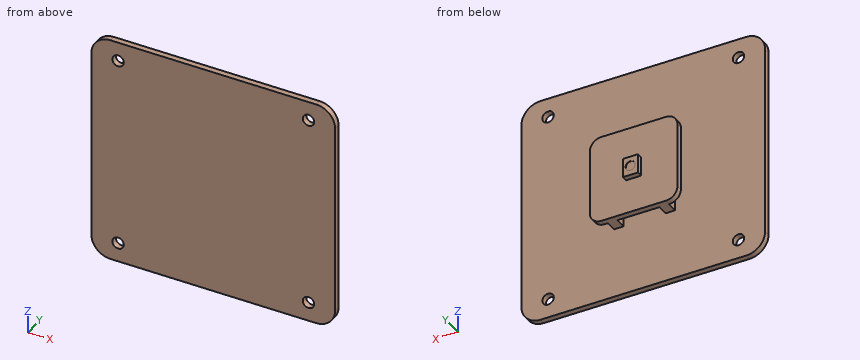
from build123d import *

# Parameters (mm, degrees)
SKETCH1_R           = 1.5
BOSS_EXTRUDE1_DEPTH = 1.6
SKETCH2_W           = 23
SKETCH2_H           = 23
BOSS_EXTRUDE2_DEPTH = 4.5
SKETCH3_W           = 4
SKETCH3_H           = 5
BOSS_EXTRUDE3_DEPTH = 1.5
SKETCH4_W           = 23
SKETCH4_H           = 2.9
CUT_EXTRUDE3_DEPTH  = 39.5
SKETCH5_W           = 2.5
SKETCH5_H           = 2.9
BOSS_EXTRUDE4_DEPTH = 23
FILLET1_R           = 3
SKETCH6_R           = 1.25
CUT_EXTRUDE4_DEPTH  = 0.1


with BuildPart() as part:
    # Sketch1 → Boss-Extrude1 (new body)
    with BuildSketch(Plane(origin=(0, 0, 0), x_dir=(1, 0, 0), z_dir=(0, 1, 0))):
        with BuildLine():
            Line((-27, -30), (27, -30))
            ThreePointArc((27, -30), (30.535533906, -28.535533906), (32, -25))
            Line((32, -25), (32, 25))
            ThreePointArc((32, 25), (30.535533906, 28.535533906), (27, 30))
            Line((27, 30), (-27, 30))
            ThreePointArc((-27, 30), (-30.535533906, 28.535533906), (-32, 25))
            Line((-32, 25), (-32, -25))
            ThreePointArc((-32, -25), (-30.535533906, -28.535533906), (-27, -30))
        make_face()
        with Locations((25, 25)):
            Circle(SKETCH1_R, mode=Mode.SUBTRACT)
        with Locations((-25, 25)):
            Circle(SKETCH1_R, mode=Mode.SUBTRACT)
        with Locations((-25, -25)):
            Circle(SKETCH1_R, mode=Mode.SUBTRACT)
        with Locations((25, -25)):
            Circle(SKETCH1_R, mode=Mode.SUBTRACT)
    extrude(amount=BOSS_EXTRUDE1_DEPTH)

    # Sketch2 → Boss-Extrude2 (add)
    with BuildSketch(Plane(origin=(0, 1.6, 0), x_dir=(1, 0, 0), z_dir=(0, 1, 0))):
        Rectangle(SKETCH2_W, SKETCH2_H)
    extrude(amount=BOSS_EXTRUDE2_DEPTH)

    # Sketch3 → Boss-Extrude3 (add)
    with BuildSketch(Plane(origin=(0, 6.1, 0), x_dir=(1, 0, 0), z_dir=(0, 1, 0))):
        Rectangle(SKETCH3_W, SKETCH3_H)
    extrude(amount=BOSS_EXTRUDE3_DEPTH)

    # Sketch4 → Cut-Extrude3 (cut)
    with BuildSketch(Plane.XY.offset(11.5)):
        with Locations((0, 3.05)):
            Rectangle(SKETCH4_W, SKETCH4_H)
    extrude(amount=-CUT_EXTRUDE3_DEPTH, mode=Mode.SUBTRACT)

    # Sketch5 → Boss-Extrude4 (add)
    with BuildSketch(Plane.XY.offset(11.5)):
        with Locations((-7.09044311, 3.05)):
            Rectangle(SKETCH5_W, SKETCH5_H)
        with Locations((6.40955689, 3.05)):
            Rectangle(SKETCH5_W, SKETCH5_H)
    extrude(amount=-BOSS_EXTRUDE4_DEPTH)

    # Fillet1
    fillet1_edges = [part.edges().sort_by_distance(p)[0] for p in [
        (11.5, 5.3, 11.5),
        (11.5, 5.3, -11.5),
        (-11.5, 5.3, -11.5),
        (-11.5, 5.3, 11.5),
    ]]
    fillet(fillet1_edges, radius=FILLET1_R)

    # Sketch6 → Cut-Extrude4 (cut)
    with BuildSketch(Plane(origin=(0, 7.6, 0), x_dir=(1, 0, 0), z_dir=(0, 1, 0))):
        Circle(SKETCH6_R)
    extrude(amount=-CUT_EXTRUDE4_DEPTH, mode=Mode.SUBTRACT)


solid = part.part
Part model, mm, in its own coordinate system. Give positions to 0.01 mm unless a question says otherwise; leave off trailing zeros. Write each loop counter-clockwise with the first axis right and the second up, starting at its lowest first coordinate (ties: lowest second). Pieces come first, ordered by that corner, then holes.
1) Cut at B-B on x = 25. Write the cut outline in (y, z), then the cut area to 3 significant figures.
Resolved:
outline: (0, -30) - (1.6, -30) - (1.6, -26.5) - (0, -26.5) - close; (0, -23.5) - (1.6, -23.5) - (1.6, 23.5) - (0, 23.5) - close; (0, 26.5) - (1.6, 26.5) - (1.6, 30) - (0, 30) - close
area: 86.4 mm2
2) Pin check, flat tips, straight feed: pin 1 (1.3 mm diameter, centred on x = 0.5, y = 4.5, fed in from -Z); pin 2 (2.5 mm diameter, centred on y = 3, z = -0.5, fed in from -X); pin 3 (2.5 mm diameter, centred on y = 3.5, z = -3.5, fed in from +X). Stop position of each tip, or through.
Resolved:
pin 1: stops at z = -11.5
pin 2: stops at x = -8.34
pin 3: stops at x = 11.5
3) Probe L1, parallel to X at y = 0.9, z = -25; L2, parallel to Z at x = -25, y = 0.9; L3, parallel to Y at x = -5.5, z = -10. List the from-to ranges inside material, lowest first.
Resolved:
L1: x = -32 to -26.5, -23.5 to 23.5, 26.5 to 32
L2: z = -30 to -26.5, -23.5 to 23.5, 26.5 to 30
L3: y = 0 to 1.6, 4.5 to 6.1
4) Cut at D-D on x = 6. Write the cut outline in (y, z), then the cut area to 4 significant figures.
Resolved:
outline: (0, -30) - (1.6, -30) - (1.6, -11.5) - (6.1, -11.5) - (6.1, 11.5) - (1.6, 11.5) - (1.6, 30) - (0, 30) - close
area: 199.5 mm2
5) Cut at C-C on z = 10.5. Write the cut outline in (x, y).
Resolved:
outline: (-32, 0) - (32, 0) - (32, 1.6) - (7.66, 1.6) - (7.66, 4.5) - (10.74, 4.5) - (10.74, 6.1) - (-10.74, 6.1) - (-10.74, 4.5) - (-8.34, 4.5) - (-8.34, 1.6) - (-32, 1.6) - close; hole (-5.84, 1.6) - (5.16, 1.6) - (5.16, 4.5) - (-5.84, 4.5) - close
6) Cut at A-A on x = -5. Write the cut outline in (y, z).
Resolved:
outline: (0, -30) - (1.6, -30) - (1.6, 30) - (0, 30) - close; (4.5, -11.5) - (6.1, -11.5) - (6.1, 11.5) - (4.5, 11.5) - close
